Geometry: see drawing. Coordinates: mm, zero at the bounding-box minimum. Round coordinates to 2 decimals unless told otherwise and drop trailing zeros. Loops run counter-clockwise (first coordinate to the right, second up) from the corner with the lowest first, then second, coordinate; pieces in that order, holes last. Notation, with made-up numbers: (-36, 32) - (-3, 32) arc R31 cw to (-3, 68) - close; hole circle Ø1 at (-11.5, 3.25). An arc over 180 degrees is marked (long way). Return JSON: item names as keys, results as strings. Group by question number.
1. Material intervals for probe 1 along Y at (x, z) = (15.25, 11.5) (1 decimal); probe 2 along Y at (x, z) = (16, 13.75) (1 decimal); probe 3 along Z at (x, y) = (20.5, 15.75) (1 decimal), sorted ascending.
2. Section B-B on z = 11.5. Return loops of the section in (x, y) (1 decimal).
3. Draft query along Y for the marked faces 1, 2, 3 and 4. Return one class per face: +Y half, -Y half, draft (parallel to the pull), parting line (faces both ways), or undercut.
4. First-contact query: pin 1 Ø10 at (x, z) = (13, 9) entering from +Y; pin 2 Ø3 at (x, y) = (20.5, 18.5) entering from -Z; pin 3 Ø1 at (x, y) = (21.5, 9.5) entering from +Z; pin 4 Ø1.5 at (x, y) = (14, 5.5) entering from +Z. Flat tips, straight axial feed; report the tip coordinate or a pass-through.
5. Section A-A on y = 11.5. Return loops of the section in (x, z) (1 decimal).
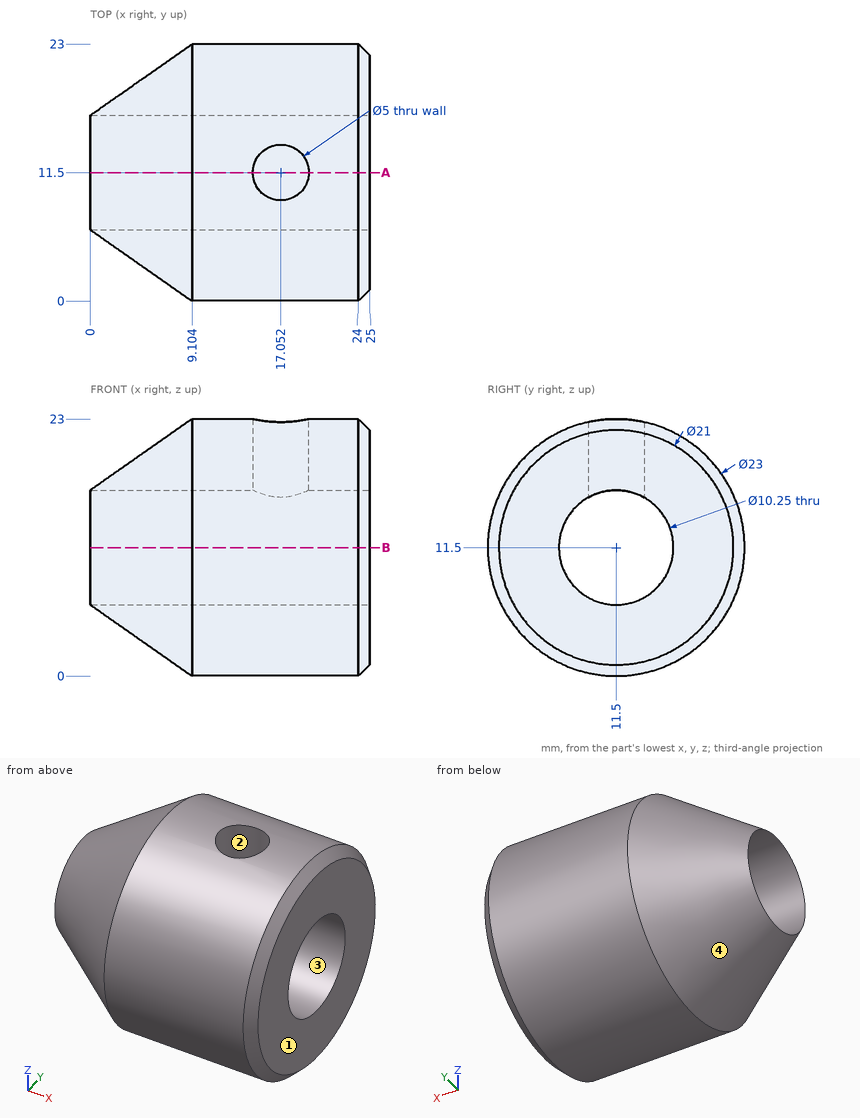
Taken from the geometry:
{
 "1": {"probe 1": "0 to 6.4, 16.6 to 23", "probe 2": "0.2 to 6.9, 16.1 to 22.8", "probe 3": "0.8 to 8.6, 14.4 to 22.2"},
 "2": {"outline": "(0, 6.4) - (9.1, 0) - (24, 0) - (25, 1) - (25, 6.4) - close; (0, 16.6) - (25, 16.6) - (25, 22) - (24, 23) - (9.1, 23) - close"},
 "3": {"face 1": "draft", "face 2": "undercut", "face 3": "undercut", "face 4": "parting line"},
 "4": {"pin 1": "y = 23", "pin 2": "z = 1.4", "pin 3": "z = 22.9", "pin 4": "z = 21.73"},
 "5": {"outline": "(0, 6.4) - (9.1, 0) - (24, 0) - (25, 1) - (25, 6.4) - close; (0, 16.6) - (14.6, 16.6) - (14.6, 23) - (9.1, 23) - close; (19.6, 16.6) - (25, 16.6) - (25, 22) - (24, 23) - (19.6, 23) - close"}
}
